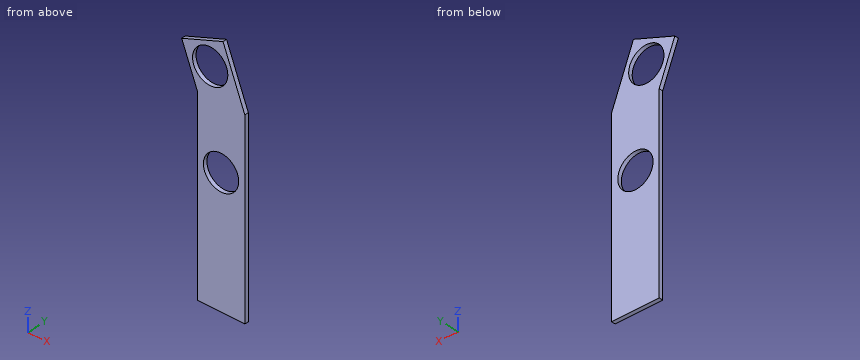
```python
from build123d import *

# Parameters (mm, degrees)
BOSS_EXTRUDE1_DEPTH = 3.175
SKETCH2_R           = 14.1605
CUT_EXTRUDE1_DEPTH  = 126.68689151
SKETCH3_R           = 14.1605
CUT_EXTRUDE2_DEPTH  = 126.68689151


with BuildPart() as part:
    # Sketch1 → Boss-Extrude1 (new body)
    with BuildSketch(Plane(origin=(0, 0, 0), x_dir=(1, 0, 0), z_dir=(0, 1, 0))):
        Polygon((-19.05, -76.2), (-31.605279538, -108.840396317), (1.584053795, -121.606827019), (19.05, -76.2), (19.05, 76.2), (-19.05, 76.2), align=None)
    extrude(amount=BOSS_EXTRUDE1_DEPTH)

    # Sketch2 → Cut-Extrude1 (cut, through all)
    with BuildSketch(Plane(origin=(0, 3.175, 0), x_dir=(1, 0, 0), z_dir=(0, 1, 0))):
        with Locations(Location((-8.732973102, -98.90341351, 0), (0, 0, 270))):
            Circle(SKETCH2_R)
    extrude(amount=-CUT_EXTRUDE1_DEPTH, mode=Mode.SUBTRACT)

    # Sketch3 → Cut-Extrude2 (cut, through all)
    with BuildSketch(Plane(origin=(0, 3.175, 0), x_dir=(1, 0, 0), z_dir=(0, 1, 0))):
        with Locations(Location((0, -25.4, 0), (0, 0, 270))):
            Circle(SKETCH3_R)
    extrude(amount=-CUT_EXTRUDE2_DEPTH, mode=Mode.SUBTRACT)


solid = part.part
```
Work out the finished part from the listing and answer in its coordinate system (mm). Round coordinates to 2 decimals unless told otherwise and drop trailing zeros. Write each loop counter-clockwise with the first axis right and the second up, starting at its lowest first coordinate (ties: lowest second). Pieces come first, ordered by that corner, then holes. Notation, with made-up numbers: (-3.75, 16) - (6.25, 16) arc R4 ccw to (6.25, 22) - close; hole circle Ø10 at (-1.5, 1). An arc over 180 degrees is marked (long way). Return JSON: item names as keys, results as strings. Group by question number.
Q1. The part is cut by section B-B on y = 0.7. Write down the section's boundary in (x, z).
Q2. The part is cut by section D-D on x = -11.5. Write down the section's boundary in (y, z) (3 decimals), then the cut area to 3 significant figures.
Q3. The part is cut by section C-C on x = 9. Write down the section's boundary in (y, z) (1 decimal).
Q4. Find the intervals of material crossed by L1, parallel to X at y = 2.2, z = 25.4; L2, parallel to Z at x = 0.5, y = 1.2; L3, parallel to X at y = 1.9, z = -18, in increasing order.
Solved:
{
 "1": {"outline": "(-31.61, 108.84) - (-19.05, 76.2) - (-19.05, -76.2) - (19.05, -76.2) - (19.05, 76.2) - (1.58, 121.61) - close; hole circle Ø28.32 at (-8.73, 98.9); hole circle Ø28.32 at (0, 25.4)"},
 "2": {"outline": "(0, -76.2) - (3.175, -76.2) - (3.175, 17.137) - (0, 17.137) - close; (0, 33.663) - (3.175, 33.663) - (3.175, 85.016) - (0, 85.016) - close; (0, 112.791) - (3.175, 112.791) - (3.175, 116.574) - (0, 116.574) - close", "area": "471 mm²"},
 "3": {"outline": "(0, -76.2) - (3.2, -76.2) - (3.2, 14.5) - (0, 14.5) - close; (0, 36.3) - (3.2, 36.3) - (3.2, 102.3) - (0, 102.3) - close"},
 "4": {"L1": "-19.05 to -14.16, 14.16 to 19.05", "L2": "-76.2 to 11.25, 39.55 to 88.17, 109.64 to 121.19", "L3": "-19.05 to 19.05"}
}
